Can you work these out from the model? Positions are in its coordinate system, mm. A direction names the side the tool comes from. Round coordinates to 2 decimals unless told otherwise and drop trailing zeros. Loops run counter-clockwise (first coordinate to the right, second up) from the corner with the lowest first, then second, coordinate; pieces in that order, holes last. Notation, with made-up numbers: (73.5, 77) -> (132.5, 77) arc R21 cw to (132.5, 92) -> close; hole circle Ø9 at (-34, -17.75). An arc over 180 degrees is marked (long way). Write item = value, one per line.
from build123d import *

# Parameters (mm, degrees)
SKETCH_W        = 50
SKETCH_H        = 126
PAD_DEPTH       = 27
THICKNESS_T     = -2
SKETCH001_W     = 51.5
SKETCH001_H     = 16.72
POCKET_DEPTH    = 50.001
SKETCH002_W     = 50
SKETCH002_H     = 15.24
PAD001_DEPTH    = 2
SKETCH003_W     = 50
SKETCH003_H     = 5
PAD002_DEPTH    = 2
SKETCH004_W     = 6
SKETCH004_H     = 15
PAD003_DEPTH    = 2
SKETCH005_W     = 6
SKETCH005_H     = 16
PAD004_DEPTH    = 2
CHAMFER_SIZE    = 1
CHAMFER001_SIZE = 1
FILLET_R        = 1
FILLET001_R     = 1


with BuildPart() as part:
    # Sketch → Pad (new body)
    with BuildSketch(Plane.XY):
        Rectangle(SKETCH_W, SKETCH_H)
    extrude(amount=PAD_DEPTH)

    # Thickness
    thickness_openings = [part.faces().sort_by_distance(p)[0] for p in [
        (0, 0, 27),
    ]]
    offset(amount=THICKNESS_T, openings=thickness_openings)

    # Sketch001 (on Face3 of Thickness) → Pocket (cut, through all)
    with BuildSketch(Plane.YZ.offset(25)):
        with Locations((-33.25, 18.64)):
            Rectangle(SKETCH001_W, SKETCH001_H)
        with Locations((33.25, 18.64)):
            Rectangle(SKETCH001_W, SKETCH001_H)
    extrude(amount=-POCKET_DEPTH, mode=Mode.SUBTRACT)

    # Sketch002 (on Face4 of Pocket) → Pad001 (join)
    with BuildSketch(Plane.XY.offset(27)):
        with Locations((0, -55.38)):
            Rectangle(SKETCH002_W, SKETCH002_H)
    extrude(amount=PAD001_DEPTH)

    # Sketch003 (on Face12 of Pad001) → Pad002 (join)
    with BuildSketch(Plane.XY.offset(27)):
        with Locations((0, 60.5)):
            Rectangle(SKETCH003_W, SKETCH003_H)
    extrude(amount=PAD002_DEPTH)

    # Sketch004 (on Face6 of Pad002) → Pad003 (join)
    with BuildSketch(Plane.XY.offset(27)):
        with Locations((22, 0)):
            Rectangle(SKETCH004_W, SKETCH004_H)
    extrude(amount=PAD003_DEPTH)

    # Sketch005 (on Face13 of Pad003) → Pad004 (join)
    with BuildSketch(Plane.XY.offset(27)):
        with Locations((-22, -0.5)):
            Rectangle(SKETCH005_W, SKETCH005_H)
    extrude(amount=PAD004_DEPTH)

    # Chamfer
    chamfer_edges = [part.edges().sort_by_distance(p)[0] for p in [
        (-19, -0.5, 29),
    ]]
    chamfer(chamfer_edges, length=CHAMFER_SIZE)

    # Chamfer001
    chamfer001_edges = [part.edges().sort_by_distance(p)[0] for p in [
        (19, 0, 29),
    ]]
    chamfer(chamfer001_edges, length=CHAMFER001_SIZE)

    # Fillet
    fillet_edges = [part.edges().sort_by_distance(p)[0] for p in [
        (0, 58, 29),
    ]]
    fillet(fillet_edges, radius=FILLET_R)

    # Fillet001
    fillet001_edges = [part.edges().sort_by_distance(p)[0] for p in [
        (0, -47.76, 29),
    ]]
    fillet(fillet001_edges, radius=FILLET001_R)


solid = part.part
1. Suppose I cut it at D-D, the plane x = -6. List the corners of the cut face in (y, z) for me, and give its area (3 significant figures).
Entries:
outline = (-63, 0) -> (63, 0) -> (63, 29) -> (59, 29) arc R1 ccw to (58, 28) -> (58, 27) -> (61, 27) -> (61, 2) -> (-61, 2) -> (-61, 27) -> (-47.76, 27) -> (-47.76, 28) arc R1 ccw to (-48.76, 29) -> (-63, 29) -> close
area = 392 mm²
2. Suppose I cut it at B-B, the plane y = -17.5. List the corners of the cut face in (x, z) for me.
Entries:
outline = (-25, 0) -> (25, 0) -> (25, 10.28) -> (23, 10.28) -> (23, 2) -> (-23, 2) -> (-23, 10.28) -> (-25, 10.28) -> close
3. I'm going to push flat-ended pins straight in: pin 1 (2 mm diameter, centred on x = 24, y = -41, fed in from +Z); pin 2 (4 mm diameter, centred on x = -1.5, y = -30, fed in from +Z). Where does each tip first touch, or does it pass through?
Entries:
pin_1 = 10.28
pin_2 = 2
4. Suppose I cut it at C-C, the plane z = 21.25. List the corners of the cut face in (x, y) for me, and give its area (3 significant figures).
Entries:
outline = (-25, -63) -> (25, -63) -> (25, -59) -> (23, -59) -> (23, -61) -> (-23, -61) -> (-23, -59) -> (-25, -59) -> close; (-25, -7.5) -> (-23, -7.5) -> (-23, 7.5) -> (-25, 7.5) -> close; (-25, 59) -> (-23, 59) -> (-23, 61) -> (23, 61) -> (23, 59) -> (25, 59) -> (25, 63) -> (-25, 63) -> close; (23, -7.5) -> (25, -7.5) -> (25, 7.5) -> (23, 7.5) -> close
area = 276 mm²
5. For faces 4 (the flat face through (-23, -1, 9)), 5 (the flat face through (23.3, -7.5, 21.6)), 6 (the flat face through (-23.4, 7.5, 21.6)), which set-ups out of +Z, -Z, +X, -X, +Y, -Y let a thin tool reach every point of the face, with its end or its side?
Entries:
face_4 = none
face_5 = +Z, +X
face_6 = +Z, +X, -X
6. Suppose I cut it at A-A, the plane z = 4.25. List the corners of the cut face in (x, y) for me.
Entries:
outline = (-25, -63) -> (25, -63) -> (25, 63) -> (-25, 63) -> close; hole (-23, -61) -> (23, -61) -> (23, 61) -> (-23, 61) -> close
7. We'd pull the mould along X, two halves only. Please class faces 1 (the flat face through (22, 0, 29)), 2 (the flat face through (21, 0, 27)), 3 (the flat face through (-25, -1, 8)): released by +X, released by -X, zero draft, split by the parting line, or undercut.
Entries:
face_1 = zero draft
face_2 = undercut
face_3 = released by -X
8. I need wall thicknesses on line 1 (X direction, y = -6, z = 27.25); line 2 (X direction, y = 4, z = 26.75); line 3 (Z direction, x = 22.5, y = -56.5). Which ranges of each line are inside material? Lowest first, please. Write a range as [from, to].
Entries:
line_1 = [-25, -19], [19, 25]
line_2 = [-25, -23], [23, 25]
line_3 = [0, 2], [27, 29]
